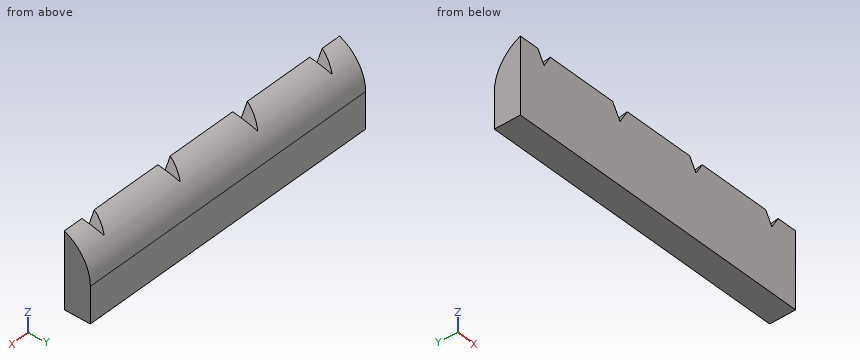
```python
from build123d import *

# Parameters (mm, degrees)
F0_W        = 36.83
F0_H        = 3.048
F1_DEPTH    = 8.89
F3_T1_DEPTH = 60.1094845304
F4_DEPTH    = 25.4


# Not quite as in the source:
# - a fillet or chamfer that OpenCascade refuses, or shapes differently, is made with other operations: its cross-section is extruded or revolved along the edge and cut away or added


with BuildPart() as f1:
    # F0 (on Top) → F1 (new body)
    with BuildSketch(Plane.XY):
        with Locations((-0.254, 1.524)):
            Rectangle(F0_W, F0_H)
    extrude(amount=F1_DEPTH)

    # F3: fillet of radius 5.08 on 1 edges, made by hand

    # F3_s2 → F3_t1 (cut)
    with BuildSketch(Plane.YZ.offset(-30.3087422652)):
        with BuildLine():
            ThreePointArc((3.048, 4.2341030939), (2.2182329348, 7.0165336861), (0, 8.89))
            Line((0, 8.89), (3.048, 8.89))
            Line((3.048, 8.89), (3.048, 4.2341030939))
        make_face()
    extrude(amount=F3_T1_DEPTH, mode=Mode.SUBTRACT)

    # F2 (on face) → F4 (cut)
    with BuildSketch(Plane.XZ):
        Polygon((-15.494, 7.4522954744), (-14.6639409051, 8.89), (-16.3240590949, 8.89), align=None)
        Polygon((-4.3572939367, 8.89), (-6.3107060633, 8.89), (-5.334, 7.1982954744), align=None)
        Polygon((5.6560590949, 8.89), (3.9959409051, 8.89), (4.826, 7.4522954744), align=None)
        Polygon((15.8160590949, 8.89), (14.1559409051, 8.89), (14.986, 7.4522954744), align=None)
    extrude(amount=-F4_DEPTH, mode=Mode.SUBTRACT)


solid = f1.part
```
Check sheet for the modelled part. Datum: model origin and axes. Units: mm. Coordinates: 2 decimals unless noted, no trailing zeros. Write each loop counter-clockwise with the first axis right and the second up, starting at its lowest first coordinate (ties: lowest second). Pieces come first, ordered by that corner, then holes. Notation, with made-up numbers: (27.5, -21) -> (65.5, -21) arc R22 ccw to (65.5, 14) -> close; hole circle Ø3 at (20.5, 64.5). An arc over 180 degrees is marked (long way). Use a Markdown table: item, result.
1. Sectioned sample at B-B (x = -2). Enter the section's corners in (y, z).
Reported:
| item | result |
|---|---|
| outline | (0, 0) -> (3.05, 0) -> (3.05, 4.23) arc R5.08 ccw to (0, 8.89) -> close |
2. Scan lines: line 1 along Y through (x, z) = (-3, 4.5); line 2 along Y through (x, z) = (-17, 6); line 3 along Z through (x, y) = (3.5, 0.4). Record each from-to range of solid material in increasing order.
Reported:
| item | result |
|---|---|
| line 1 | y = 0 to 3.04 |
| line 2 | y = 0 to 2.73 |
| line 3 | z = 0 to 8.69 |
3. Sectioned sample at C-C (z = 6.5). Enter the section's corners in (x, y).
Reported:
| item | result |
|---|---|
| outline | (-18.67, 0) -> (18.16, 0) -> (18.16, 2.51) -> (-18.67, 2.51) -> close |
4. Sectioned sample at A-A (y = 0.95). Enter the section's corners in (x, z).
Reported:
| item | result |
|---|---|
| outline | (-18.67, 0) -> (18.16, 0) -> (18.16, 8.35) -> (15.5, 8.35) -> (14.99, 7.45) -> (14.47, 8.35) -> (5.34, 8.35) -> (4.83, 7.45) -> (4.31, 8.35) -> (-4.67, 8.35) -> (-5.33, 7.2) -> (-6, 8.35) -> (-14.98, 8.35) -> (-15.49, 7.45) -> (-16.01, 8.35) -> (-18.67, 8.35) -> close |
